```python
from build123d import *

# Parameters (mm, degrees)
PAD_DEPTH = 2


with BuildPart() as part:
    # Sketch → Pad (new body)
    with BuildSketch(Plane.XY):
        with BuildLine():
            Line((-55.5, 20), (55.5, 20))
            Line((55.5, 20), (55.5, -4))
            Line((55.5, -4), (34.5, -4))
            Line((34.5, 4.877501), (34.5, -4))
            ThreePointArc((34.5, 4.877501), (32, 12), (29.5, 4.877501))
            Line((29.5, -4), (29.5, 4.877501))
            Line((29.5, -4), (-29.5, -4))
            Line((-29.5, 4.877501), (-29.5, -4))
            ThreePointArc((-29.5, 4.877501), (-32, 12), (-34.5, 4.877501))
            Line((-34.5, -4), (-34.5, 4.877501))
            Line((-34.5, -4), (-55.5, -4))
            Line((-55.5, -4), (-55.5, 20))
        make_face()
    extrude(amount=PAD_DEPTH)


solid = part.part
```
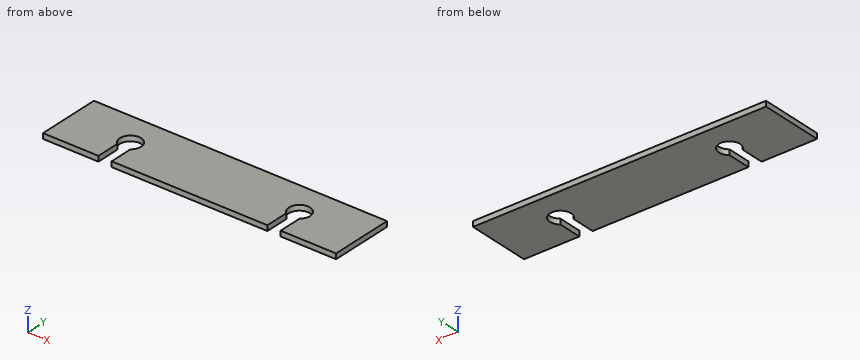
CAD build for the part. Positions are in the model's coordinates, mm. Give positions to 0.01 mm unless a question says otherwise; leave off trailing zeros. Order: outer loops, then holes, each group sorted by start corner. A loop starts at its lowest first (then second) coordinate and runs counter-clockwise, first axis right, second up.
(1) Saw through at A-A, the plane y = 2. Give the cut face in (x, z).
(2) Saw through at C-C, the plane y = 8. Give the cut face in (x, z).
(3) Drill centre lines: L1, parallel to X at y = 8, z = 1.35; L2, parallel to X at y = 3.25, z = 1; L3, parallel to Y at x = 32, z = 1.55. Where is each one in solid material? Low to high.
(4) Saw through at B-B, the plane z = 1.55. Give the cut face in (x, y), then the cut area to 3 significant figures.
(5) Saw through at D-D, the plane x = -32. Give the cut face in (y, z).
(6) Flat gauge pin, fed straight in: pin 1 (6.5 mm diameter, centred on x = -32, y = 8, fed in from -Z). Where does the tip first touch, or does it go through?
Results found:
1. outline: (-55.5, 0) - (-34.5, 0) - (-34.5, 2) - (-55.5, 2) - close; (-29.5, 0) - (29.5, 0) - (29.5, 2) - (-29.5, 2) - close; (34.5, 0) - (55.5, 0) - (55.5, 2) - (34.5, 2) - close
2. outline: (-55.5, 0) - (-36, 0) - (-36, 2) - (-55.5, 2) - close; (-28, 0) - (28, 0) - (28, 2) - (-28, 2) - close; (36, 0) - (55.5, 0) - (55.5, 2) - (36, 2) - close
3. L1: x = -55.5 to -36, -28 to 28, 36 to 55.5
3. L2: x = -55.5 to -34.5, -29.5 to 29.5, 34.5 to 55.5
3. L3: y = 12 to 20
4. outline: (-55.5, -4) - (-34.5, -4) - (-34.5, 4.88) arc R4 cw (long way) to (-29.5, 4.88) - (-29.5, -4) - (29.5, -4) - (29.5, 4.88) arc R4 cw (long way) to (34.5, 4.88) - (34.5, -4) - (55.5, -4) - (55.5, 20) - (-55.5, 20) - close
4. area: 2,480 mm2
5. outline: (12, 0) - (20, 0) - (20, 2) - (12, 2) - close
6. pin 1: passes through
